Read the model definition and answer for the solid it produces. Units are mm, in the model's axes. A direction names the side the tool comes from. Round coordinates to 2 decimals unless told otherwise and drop trailing zeros. Write each loop counter-clockwise with the first axis right and the second up, starting at its lowest first coordinate (ties: lowest second). Pieces come first, ordered by that corner, then holes. Notation, with made-up numbers: (27, -33) - (77, -33) arc R18 ccw to (77, -25) - close; hole circle Ø5 at (27, -19.75). An arc over 180 degrees is marked (long way). One line per item, written item: value. Start each with the question number.
(1) A cutting plane is placed at B-B, the plane y = 0. Determine the outline of the cut face in (x, z).
(2) The mould has two halves that part along Y. Classify faces 1 (the face through (3.226, 0.526, 6.331)), 2 (the face through (5, 1.2, -5.04)), 3 (the face through (3, 0, 11)): +Y half, -Y half, draft (parallel to the pull), parting line (faces both ways), or undercut.
(3) A cutting plane is placed at D-D, the plane y = 3.75. Determine the outline of the cut face in (x, z).
(4) A cutting plane is placed at C-C, the plane x = 3.75. Determine the outline of the cut face in (y, z).
(5) For faces 4 (the face through (10.67, -4.88, 1.08)), 5 (the face through (3.226, 0.526, -9.669)), determine the directions among +Z, -Z, +X, -X, +Y, -Y from which every point of the face is accessible in a straight line to the end or side of a thin tool.
(6) Find the intervals of material crossed by L1, parallel to Y at x = 3.5, z = 8; L2, parallel to Y at x = 11.75, z = 0; L3, parallel to Z at x = 12.5, y = 0.5, in increasing order.
(7) Flat-ended cylindrical pins translate along their axes: pin 1 Ø1 at (y, z) = (-2, 7) entering from +X; pin 2 Ø1.5 at (x, z) = (10, -3.5) entering from -Y; pin 3 Ø5 at (x, y) = (9.5, 1) entering from +Z. Find the tip coordinate at first contact, or state that the pin passes through.
(8) A cutting plane is placed at A-A, the plane z = 0. Determine the outline of the cut face in (x, y).
from build123d import *

# Parameters (mm, degrees)
SKETCH_1_R          = 5
SKETCH_1_R_2        = 4
EXTRUDE_1_DEPTH     = 1.5
SKETCH_2_R          = 4
SKETCH_2_R_2        = 1.75
EXTRUDE_2_DEPTH     = 3.5
SKETCH_3_R          = 5
SKETCH_3_R_2        = 4
EXTRUDE_3_DEPTH     = 11.5
SKETCH_4_R          = 5
CUT_EXTRUDE_1_DEPTH = 1.5


with BuildPart() as part:
    # 草图1 → 凸台-拉伸1 (new body)
    with BuildSketch(Plane(origin=(0, 0, 0), x_dir=(0, 0, -1), z_dir=(1, 0, 0))):
        Circle(SKETCH_1_R)
        Circle(SKETCH_1_R_2, mode=Mode.SUBTRACT)
    extrude(amount=EXTRUDE_1_DEPTH)

    # 草图2 → 凸台-拉伸2 (add)
    with BuildSketch(Plane(origin=(1.5, 0, 0), x_dir=(0, 0, -1), z_dir=(1, 0, 0))):
        with BuildLine():
            Line((-9.746281342, 5.1), (9.746281342, 5.1))
            ThreePointArc((9.746281342, 5.1), (11, 0), (9.746281342, -5.1))
            Line((9.746281342, -5.1), (-9.746281342, -5.1))
            ThreePointArc((-9.746281342, -5.1), (-11, 0), (-9.746281342, 5.1))
        make_face()
        Circle(SKETCH_2_R, mode=Mode.SUBTRACT)
        with Locations((-8, 0)):
            Circle(SKETCH_2_R_2, mode=Mode.SUBTRACT)
        with Locations((8, 0)):
            Circle(SKETCH_2_R_2, mode=Mode.SUBTRACT)
    extrude(amount=EXTRUDE_2_DEPTH)

    # 草图3 → 凸台-拉伸3 (add)
    with BuildSketch(Plane(origin=(5, 0, 0), x_dir=(0, 0, -1), z_dir=(1, 0, 0))):
        Circle(SKETCH_3_R)
        Circle(SKETCH_3_R_2, mode=Mode.SUBTRACT)
    extrude(amount=EXTRUDE_3_DEPTH)

    # 草图4 → 切除-拉伸1 (cut)
    with BuildSketch(Plane.ZY):
        with Locations(Location((0, 0, 0), (0, 0, 180))):
            Circle(SKETCH_4_R)
    extrude(amount=-CUT_EXTRUDE_1_DEPTH, mode=Mode.SUBTRACT)


solid = part.part
Here are the results:
1. outline: (1.5, -11) - (5, -11) - (5, -9.75) - (1.5, -9.75) - close; (1.5, -6.25) - (5, -6.25) - (5, -5) - (16.5, -5) - (16.5, -4) - (1.5, -4) - close; (1.5, 4) - (16.5, 4) - (16.5, 5) - (5, 5) - (5, 6.25) - (1.5, 6.25) - close; (1.5, 9.75) - (5, 9.75) - (5, 11) - (1.5, 11) - close
2. face 1: undercut
2. face 2: draft
2. face 3: parting line
3. outline: (1.5, -10.34) - (5, -10.34) - (5, -3.31) - (16.5, -3.31) - (16.5, -1.39) - (1.5, -1.39) - close; (1.5, 1.39) - (16.5, 1.39) - (16.5, 3.31) - (5, 3.31) - (5, 10.34) - (1.5, 10.34) - close
4. outline: (-5.1, -9.75) arc R11 ccw to (5.1, -9.75) - (5.1, 9.75) arc R11 ccw to (-5.1, 9.75) - close; hole circle Ø8 at (0, 0); hole circle Ø3.5 at (0, -8); hole circle Ø3.5 at (0, 8)
5. face 4: +X
5. face 5: +X, -X
6. L1: -5.1 to -1.75, 1.75 to 5.1
6. L2: -5 to -4, 4 to 5
6. L3: -4.97 to -3.97, 3.97 to 4.97
7. pin 1: x = 5
7. pin 2: y = -4.18
7. pin 3: z = 5
8. outline: (1.5, -5.1) - (5, -5.1) - (5, -5) - (16.5, -5) - (16.5, -4) - (1.5, -4) - close; (1.5, 4) - (16.5, 4) - (16.5, 5) - (5, 5) - (5, 5.1) - (1.5, 5.1) - close
